Part model, mm, in its own coordinate system. Face numbers are marked on the shaded views. A direction names the side the tool comes from. Round coordinates to 2 decimals unless told otherwise and drop trailing zeros. Loops run counter-clockwise (first coordinate to the right, second up) from the corner with the lowest first, then second, coordinate; pieces in that order, holes last. Notation, with made-up numbers: M 57.25,4 L 107.25,4 A25 ccw 107.25,31 Z; hole C -30.5,23.25 d10. An arc over 180 degrees is marked long. Put each result on its own line as item: value. Start each with the question number.
1) Slice it at D-D on y = 10. Give the cut face in (x, z).
2) Probe line 1 along Z through (x, y) = (0, 1.95); line 2 along Y through (x, z) = (16, -38.35); line 3 along X through (y, z) = (1.85, 30). List the from-to ranges inside material, lowest first.
3) Slice it at B-B on x = 0. Give the cut face in (y, z), then the cut area to 3 significant figures.
4) Slice it at A-A on z = 30. Give the cut face in (x, y), then the cut area to 3 significant figures.
5) Drop flat-ended pins along their axis: pin 1 Ø8 at (x, z) = (0, 30) entering from -Y; pin 2 Ø6 at (x, z) = (5, 25) entering from +Y; pin 3 Ø0.9 at (y, z) = (1, 15.5) entering from +X; pin 4 Ø6 at (x, y) = (14.5, 9.5) entering from +Z. Give the stop position or say it passes through.
6) Which spindle directions (+Z, -Z, +X, -X, +Y, -Y) get a long thin tool onto all of the face, cutting with end or side? Do the marked faces 1 and 2. Say none if no direction does.
7) Slice it at C-C on y = 2.25. Give the cut face in (x, z).
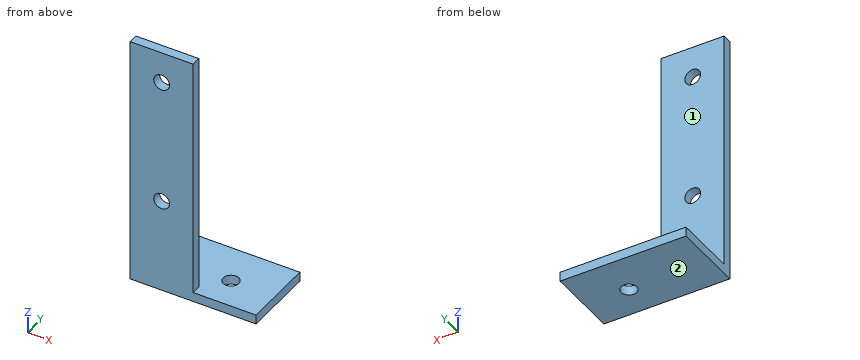
```python
from build123d import *

# Parameters (mm, degrees)
SKETCH1_W           = 20
SKETCH1_H           = 80
SKETCH1_R           = 2.5
BOSS_EXTRUDE1_DEPTH = 3
SKETCH2_W           = 20
SKETCH2_H           = 3
BOSS_EXTRUDE2_DEPTH = 20
SKETCH8_W           = 3
SKETCH8_H           = 23
BOSS_EXTRUDE5_DEPTH = 20
SKETCH9_R           = 2.5
CUT_EXTRUDE3_DEPTH  = 20


with BuildPart() as part:
    # Sketch1 → Boss-Extrude1 (new body)
    with BuildSketch(Plane(origin=(0, 0, 0), x_dir=(1, 0, 0), z_dir=(0, 1, 0))):
        Rectangle(SKETCH1_W, SKETCH1_H)
        with Locations((0, -30)):
            Circle(SKETCH1_R, mode=Mode.SUBTRACT)
        with Locations((0, 10)):
            Circle(SKETCH1_R, mode=Mode.SUBTRACT)
    extrude(amount=BOSS_EXTRUDE1_DEPTH)

    # Sketch2 → Boss-Extrude2 (add)
    with BuildSketch(Plane(origin=(0, 3, 0), x_dir=(1, 0, 0), z_dir=(0, 1, 0))):
        with Locations((0, 38.5)):
            Rectangle(SKETCH2_W, SKETCH2_H)
    extrude(amount=BOSS_EXTRUDE2_DEPTH)

    # Sketch8 → Boss-Extrude5 (add)
    with BuildSketch(Plane(origin=(10, 0, 0), x_dir=(0, 0, -1), z_dir=(1, 0, 0))):
        with Locations((38.5, 11.5)):
            Rectangle(SKETCH8_W, SKETCH8_H)
    extrude(amount=BOSS_EXTRUDE5_DEPTH)

    # Sketch9 → Cut-Extrude3 (cut)
    with BuildSketch(Plane(origin=(0, 0, -40), x_dir=(-1, 0, 0), z_dir=(0, 0, -1))):
        with Locations((-16, 10)):
            Circle(SKETCH9_R)
    extrude(amount=-CUT_EXTRUDE3_DEPTH, mode=Mode.SUBTRACT)


solid = part.part
```
Recorded:
1. outline: M -10,-40 L 13.5,-40 L 13.5,-37 L -10,-37 Z; M 18.5,-40 L 30,-40 L 30,-37 L 18.5,-37 Z
2. line 1: z = -40 to -12.5, -7.5 to 27.5, 32.5 to 40
2. line 2: y = 0 to 7.5, 12.5 to 23
2. line 3: x = -10 to -2.5, 2.5 to 10
3. outline: M 0,-40 L 23,-40 L 23,-37 L 3,-37 L 3,-12.5 L 0,-12.5 Z; M 0,-7.5 L 3,-7.5 L 3,27.5 L 0,27.5 Z; M 0,32.5 L 3,32.5 L 3,40 L 0,40 Z
3. area: 270 mm2
4. outline: M -10,0 L -2.5,0 L -2.5,3 L -10,3 Z; M 2.5,0 L 10,0 L 10,3 L 2.5,3 Z
4. area: 45.0 mm2
5. pin 1: stops at y = 0
5. pin 2: stops at y = 3
5. pin 3: stops at x = 10
5. pin 4: stops at z = -37
6. face 1: +Z, +X, -X, +Y
6. face 2: -Z, +X, -X, +Y, -Y
7. outline: M -10,-40 L 30,-40 L 30,-37 L 10,-37 L 10,40 L -10,40 Z; hole C 0,-10 d5; hole C 0,30 d5
